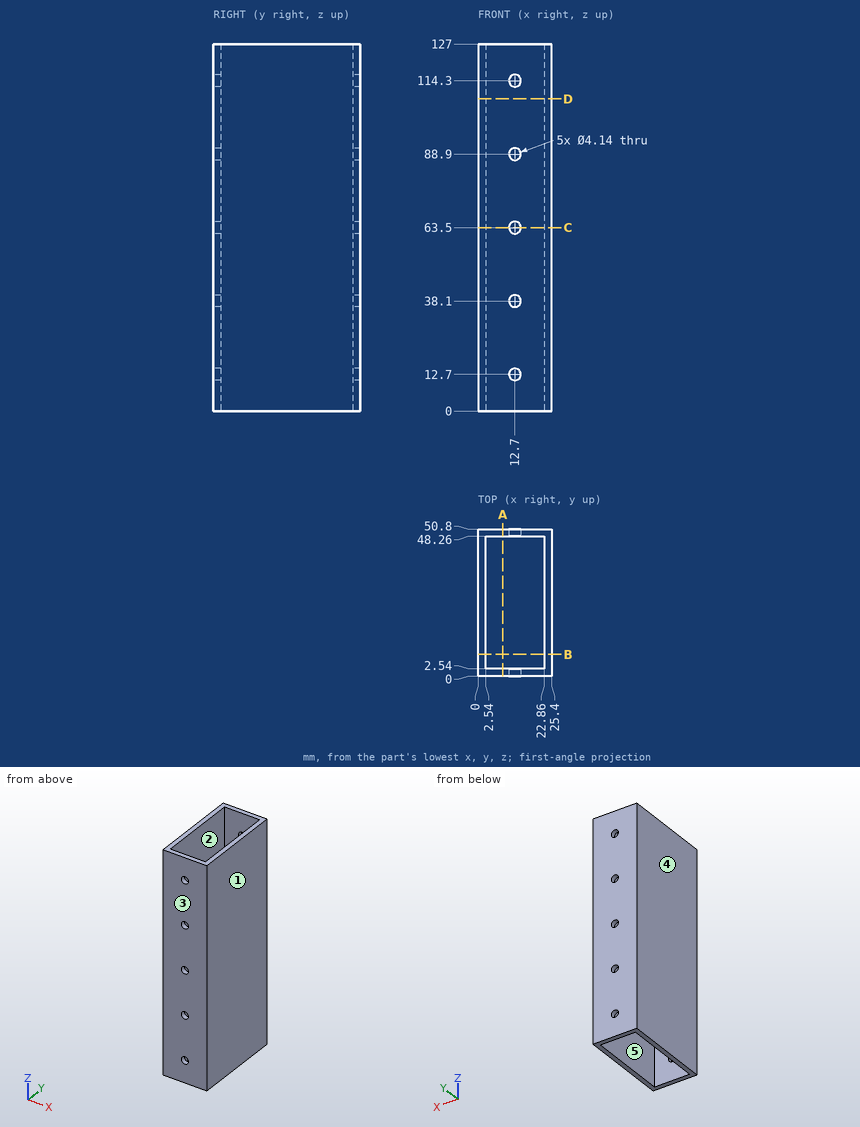
Job drawing, mm, ordinate dimensions from the low corner. One solid piece. A direction names the side the tool comes from. Round coordinates to 2 decimals unless told otherwise and drop trailing zeros. Write each loop counter-clockwise with the first axis right and the second up, starting at its lowest first coordinate (ties: lowest second). Pieces come first, ordered by that corner, then holes. Notation, with made-up numbers: (81.25, 6.25) -> (108.25, 6.25) arc R21 ccw to (108.25, 14.25) -> close; hole circle Ø5 at (58.5, 61.25). An arc over 180 degrees is marked (long way). Answer as a JSON object with one key per item and string values.
(1) Band-saw the part on C-C, the plane z = 63.5. List the corners of the cut face in (x, y), then the cut area to 3 significant figures.
Reported:
{"outline": "(0, 0) -> (10.63, 0) -> (10.63, 2.54) -> (2.54, 2.54) -> (2.54, 48.26) -> (10.63, 48.26) -> (10.63, 50.8) -> (0, 50.8) -> close; (14.77, 0) -> (25.4, 0) -> (25.4, 50.8) -> (14.77, 50.8) -> (14.77, 48.26) -> (22.86, 48.26) -> (22.86, 2.54) -> (14.77, 2.54) -> close", "area": "340 mm^2"}
(2) Band-saw the part on A-A, the plane x = 8.5. List the corners of the cut face in (y, z), then the cut area to 3 significant figures.
Reported:
{"outline": "(0, 0) -> (2.54, 0) -> (2.54, 127) -> (0, 127) -> close; (48.26, 0) -> (50.8, 0) -> (50.8, 127) -> (48.26, 127) -> close", "area": "645 mm^2"}
(3) Two-plate mould, pull along Y, no slides. Class the marked faces 1, 2 and 3: +Y half, -Y half, draft (parallel to the pull), parting line (faces both ways), or undercut.
Reported:
{"face 1": "draft", "face 2": "undercut", "face 3": "-Y half"}
(4) Which spindle directions (+Z, -Z, +X, -X, +Y, -Y) get a long thin tool onto all of the face, cutting with end or side? Do the marked faces 4 and 5. Say none if no direction does.
Reported:
{"face 4": "+Z, -Z, -X, +Y, -Y", "face 5": "+Z, -Z"}
(5) Band-saw the part on D-D, the plane z = 108. List the corners of the cut face in (x, y).
Reported:
{"outline": "(0, 0) -> (25.4, 0) -> (25.4, 50.8) -> (0, 50.8) -> close; hole (2.54, 2.54) -> (22.86, 2.54) -> (22.86, 48.26) -> (2.54, 48.26) -> close"}
(6) Probe probe 1 along Z at (x, y) = (12.7, 0.9); probe 2 along Y at (x, z) = (18.5, 65); probe 3 along X at (y, z) = (31.5, 60). List the from-to ranges inside material, lowest first. Write a range as [from, to].
Reported:
{"probe 1": "z = [0, 10.63], [14.77, 36.03], [40.17, 61.43], [65.57, 86.83], [90.97, 112.23], [116.37, 127]", "probe 2": "y = [0, 2.54], [48.26, 50.8]", "probe 3": "x = [0, 2.54], [22.86, 25.4]"}
(7) Band-saw the part on B-B, the plane y = 7.5. List the corners of the cut face in (x, z), then the cut area to 3 significant figures.
Reported:
{"outline": "(0, 0) -> (2.54, 0) -> (2.54, 127) -> (0, 127) -> close; (22.86, 0) -> (25.4, 0) -> (25.4, 127) -> (22.86, 127) -> close", "area": "645 mm^2"}
(8) Pin check, flat tip, straight feed: P1, Ø6, axis at x = 4.5, y = 33, coming from the +Z side. Stop position of the tip, or through.
Reported:
{"P1": "stops at z = 127"}
